```python
from build123d import *

# Parameters (mm, degrees)
F1_DEPTH = 2.5
F2_W     = 8.188494
F2_H     = 2.5
F3_DEPTH = 0.75
F4_W     = 1.2
F4_H     = 2.5
F5_DEPTH = 0.75
F6_R     = 0.3
F7_DEPTH = 5


with BuildPart() as f1:
    # F0 (on Top) → F1 (new body)
    with BuildSketch(Plane.XY):
        Polygon((5, -0.6), (5, 2.5), (-5, 2.5), (-5, -2.5), (5, -2.5), (5, -1.6), (4.5, -1.6), (4.5, -0.6), align=None)
    extrude(amount=F1_DEPTH)

    # F2 (on face) → F3 (join)
    with BuildSketch(Plane.XZ.offset(2.5)):
        with Locations((-0.905753, 1.25)):
            Rectangle(F2_W, F2_H)
    extrude(amount=F3_DEPTH)

    # F4 (on face) → F5 (join)
    with BuildSketch(Plane.XZ.offset(3.25)):
        with Locations((-1.4, 1.25)):
            Rectangle(F4_W, F4_H)
        with Locations((-0.2, 1.25)):
            Rectangle(F4_W, F4_H)
    extrude(amount=F5_DEPTH)

    # F6 (on face) → F7 (join)
    with BuildSketch(Plane(origin=(0, 2.5, 0), x_dir=(-1, 0, 0), z_dir=(0, 1, 0))):
        with Locations((2.54, 1.25)):
            Circle(F6_R)
        with Locations((0, 1.25)):
            Circle(F6_R)
        with Locations((-2.54, 1.25)):
            Circle(F6_R)
    extrude(amount=F7_DEPTH)


solid = f1.part
```
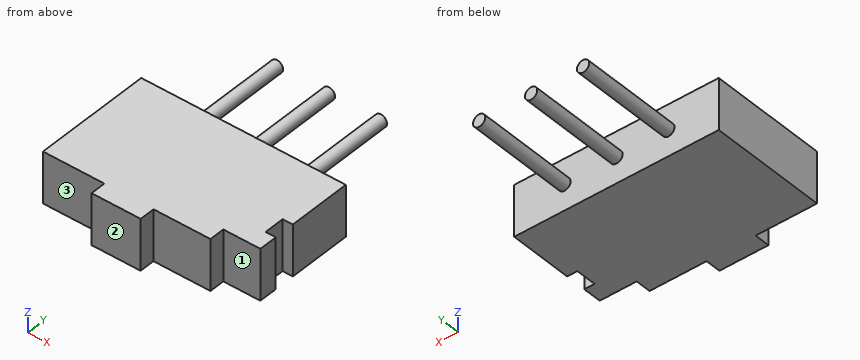
CAD build for the part. Positions are in the model's coordinates, mm. Face numbers are marked on the shaded views. A direction names the side the tool comes from. Round coordinates to 2 decimals unless told otherwise and drop trailing zeros. Order: outer loops, then holes, each group sorted by start corner. A loop starts at its lowest first (then second) coordinate and runs counter-clockwise, first axis right, second up.
Q1. Which spindle directions (+Z, -Z, +X, -X, +Y, -Y) get a long thin tool onto all of the face, cutting with end or side? Do the marked faces 1, 2 and 3. Say none if no direction does.
Q2. Slice it at C-C (y = 4). Write the cut outline in (x, z), and give its area (3 significant figures).
Q3. Slice it at D-D (z = 1.25). Write the cut outline in (x, y), and give its area (3 significant figures).
Q4. Slice it at A-A (x = 2.54). Write the cut outline in (y, z), and give its area (3 significant figures).
Q5. Slice it at B-B (z = 0.25). Write the cut outline in (x, y).
Q6. Drop flat-ended pins along their axis: pin 1 (6 mm diameter, centred on x = 0.5, y = 6, fed in from +Z); pin 2 (1 mm diameter, centred on x = 0, y = 4.5, fed in from -Z); pin 3 (1.5 mm diameter, centred on y = 3.5, z = 1, fed in from -X). Give the stop position or say it passes through.
Q7. Wall check: L1, parallel to Y at x = -0.75, z = 1.75; L2, parallel to X at y = -1.5, z = 0.55; L3, parallel to Y at x = -3.5, z = 1.85. Give the ranges that are in metal, low to high.
Results below:
1. face 1: +Z, -Z, +X, -Y
1. face 2: +Z, -Z, +X, -X, -Y
1. face 3: +Z, -Z, -X, -Y
2. outline: circle Ø0.6 at (-2.54, 1.25); circle Ø0.6 at (0, 1.25); circle Ø0.6 at (2.54, 1.25)
2. area: 0.848 mm2
3. outline: (-5, -3.25) - (-2, -3.25) - (-2, -4) - (0.4, -4) - (0.4, -3.25) - (3.19, -3.25) - (3.19, -2.5) - (5, -2.5) - (5, -1.6) - (4.5, -1.6) - (4.5, -0.6) - (5, -0.6) - (5, 2.5) - (2.84, 2.5) - (2.84, 7.5) - (2.24, 7.5) - (2.24, 2.5) - (0.3, 2.5) - (0.3, 7.5) - (-0.3, 7.5) - (-0.3, 2.5) - (-2.24, 2.5) - (-2.24, 7.5) - (-2.84, 7.5) - (-2.84, 2.5) - (-5, 2.5) - close
3. area: 66.4 mm2
4. outline: (-3.25, 0) - (2.5, 0) - (2.5, 0.95) - (7.5, 0.95) - (7.5, 1.55) - (2.5, 1.55) - (2.5, 2.5) - (-3.25, 2.5) - close
4. area: 17.4 mm2
5. outline: (-5, -3.25) - (-2, -3.25) - (-2, -4) - (0.4, -4) - (0.4, -3.25) - (3.19, -3.25) - (3.19, -2.5) - (5, -2.5) - (5, -1.6) - (4.5, -1.6) - (4.5, -0.6) - (5, -0.6) - (5, 2.5) - (-5, 2.5) - close
6. pin 1: stops at z = 1.55
6. pin 2: stops at z = 0.95
6. pin 3: stops at x = -2.84
7. L1: y = -4 to 2.5
7. L2: x = -5 to 4.5
7. L3: y = -3.25 to 2.5
